from build123d import *

# Parameters (mm, degrees)
SKETCH1_W                      = 300
SKETCH1_H                      = 300
BOSS_EXTRUDE1_DEPTH            = 175
SHELL1_T                       = -10
CUT_EXTRUDE5_DEPTH             = 50
CUT_EXTRUDE6_START             = -50
CUT_EXTRUDE6_DEPTH             = 50
CUT_EXTRUDE7_REACH             = 380.319
SKETCH8_W                      = 150
SKETCH8_H                      = 20
CUT_EXTRUDE7_DIRECTION_2_DEPTH = 379.318648761


with BuildPart() as part:
    # Sketch1 → Boss-Extrude1 (new body)
    with BuildSketch(Plane(origin=(0, 0, 0), x_dir=(1, 0, 0), z_dir=(0, 1, 0))):
        Rectangle(SKETCH1_W, SKETCH1_H)
    extrude(amount=BOSS_EXTRUDE1_DEPTH)

    # Shell1
    shell1_openings = [part.faces().sort_by_distance(p)[0] for p in [
        (0, 175, 0),
    ]]
    offset(amount=SHELL1_T, openings=shell1_openings, kind=Kind.INTERSECTION)

    # Sketch4 → Cut-Extrude5 (cut)
    with BuildSketch(Plane.XY.offset(150)):
        with BuildLine():
            Line((0, 0), (75, 0))
            Line((75, 0), (75, 50))
            ThreePointArc((75, 50), (83.786796564, 71.213203436), (105, 80))
            Line((105, 80), (150, 80))
            Line((150, 80), (150, -5))
            Line((150, -5), (-150, -5))
            Line((-150, -5), (-150, 80))
            Line((-150, 80), (-105, 80))
            ThreePointArc((-105, 80), (-83.786796564, 71.213203436), (-75, 50))
            Line((-75, 50), (-75, 0))
            Line((-75, 0), (0, 0))
        make_face()
    extrude(amount=-CUT_EXTRUDE5_DEPTH, mode=Mode.SUBTRACT)

    # Sketch7 → Cut-Extrude6 (cut)
    with BuildSketch(Plane(origin=(0, 0, -150), x_dir=(-1, 0, 0), z_dir=(0, 0, -1)).offset(CUT_EXTRUDE6_START)):
        with BuildLine():
            Line((0, 0), (75, 0))
            Line((75, 0), (75, 50))
            ThreePointArc((75, 50), (83.786796564, 71.213203436), (105, 80))
            Line((105, 80), (150, 80))
            Line((150, 80), (150, -5))
            Line((150, -5), (-150, -5))
            Line((-150, -5), (-150, 80))
            Line((-150, 80), (-105, 80))
            ThreePointArc((-105, 80), (-83.786796564, 71.213203436), (-75, 50))
            Line((-75, 50), (-75, 0))
            Line((-75, 0), (0, 0))
        make_face()
    extrude(amount=CUT_EXTRUDE6_DEPTH, mode=Mode.SUBTRACT)

    # Sketch8 → Cut-Extrude7 (cut, up to next)
    with BuildSketch(Plane(origin=(150, 0, 0), x_dir=(0, 0, -1), z_dir=(1, 0, 0)), mode=Mode.PRIVATE) as cut_extrude7_sk1:
        with Locations((0, 100)):
            Rectangle(SKETCH8_W, SKETCH8_H)
    cut_extrude7_tool1 = extrude(cut_extrude7_sk1.sketch, amount=-CUT_EXTRUDE7_REACH, mode=Mode.PRIVATE) & part.part
    add(cut_extrude7_tool1.solids().sort_by_distance((150, 100, 0))[0], mode=Mode.SUBTRACT)

    # Sketch8 → Cut-Extrude7 direction 2 (cut)
    with BuildSketch(Plane(origin=(150, 0, 0), x_dir=(0, 0, -1), z_dir=(1, 0, 0))):
        with Locations((0, 100)):
            Rectangle(SKETCH8_W, SKETCH8_H)
    extrude(amount=CUT_EXTRUDE7_DIRECTION_2_DEPTH, mode=Mode.SUBTRACT)


solid = part.part
Source: CAD feature listing. Evaluate the final solid. Frame: model axes, mm. A direction names the side the tool comes from. Give positions to 0.01 mm unless a question says otherwise; leave off trailing zeros. Order: outer loops, then holes, each group sorted by start corner. A loop starts at its lowest first (then second) coordinate and runs counter-clockwise, first axis right, second up. Notation, with made-up numbers: (32, 53) -> (42, 53) arc R6 ccw to (42, 58) -> close; hole circle Ø9 at (46.5, 65.25). An arc over 180 degrees is marked (long way). Use a Markdown table: item, result.
1) Section query B-B, the plane y = 31.5. Return the cut outline in (x, z).
Answer list:
| item | result |
|---|---|
| outline | (-150, -100) -> (-140, -100) -> (-140, 100) -> (-150, 100) -> close; (-75, -150) -> (75, -150) -> (75, -140) -> (-75, -140) -> close; (-75, 140) -> (75, 140) -> (75, 150) -> (-75, 150) -> close; (140, -100) -> (150, -100) -> (150, 100) -> (140, 100) -> close |
2) Reachability of faces 1 (the flat face through (-2, 110, -140)), 2 (the flat face through (145, 110, 1)), 3 (the flat face through (142, 80, 136)) from +Z, -Z, +X, -X, +Y, -Y: full face, straight path, thin tool, end or side. Return the list, or none.
Answer list:
| item | result |
|---|---|
| face 1 | +Y |
| face 2 | +X |
| face 3 | +Z, +X, -Y |
3) Contact query for flat-ended pins moving along their axis: P1, Ø13.5, axis at x = 136, z = -135.5, coming from the -Y side; P2, Ø3, axis at x = 33, z = 47, coming from the +Y side. Output: stop coordinate, or through.
Answer list:
| item | result |
|---|---|
| P1 | y = 80 |
| P2 | y = 10 |
4) Section query D-D, the plane x = 128.5. Return the cut outline in (y, z).
Answer list:
| item | result |
|---|---|
| outline | (0, -100) -> (10, -100) -> (10, 100) -> (0, 100) -> close; (80, -150) -> (175, -150) -> (175, -140) -> (80, -140) -> close; (80, 140) -> (175, 140) -> (175, 150) -> (80, 150) -> close |
5) Section query C-C, the plane z = 1.5. Return the cut outline in (x, y).
Answer list:
| item | result |
|---|---|
| outline | (-150, 0) -> (150, 0) -> (150, 90) -> (140, 90) -> (140, 10) -> (-140, 10) -> (-140, 175) -> (-150, 175) -> close; (140, 110) -> (150, 110) -> (150, 175) -> (140, 175) -> close |
6) Section query A-A, the plane z = -120. Return the cut outline in (x, y).
Answer list:
| item | result |
|---|---|
| outline | (-150, 80) -> (-140, 80) -> (-140, 175) -> (-150, 175) -> close; (-75, 0) -> (75, 0) -> (75, 10) -> (-75, 10) -> close; (140, 80) -> (150, 80) -> (150, 175) -> (140, 175) -> close |
7) Mould query, pull axis Z, two halves, no side actions, for faces 4 (the flat face through (75, 8, 136)), 5 (the flat face through (-2, 10, -2)), 6 (the flat face through (-143, 25, 100)), 7 (the flat face through (-2, 106, -150)). Classes: +Z half, -Z half, draft (parallel to the pull), parting line (faces both ways), or undercut.
Answer list:
| item | result |
|---|---|
| face 4 | draft |
| face 5 | undercut |
| face 6 | +Z half |
| face 7 | -Z half |
8) Ray query, line 1 along Z through (x, y) = (72, 136); line 2 along Y through (x, z) = (-117.5, -25). Return the intervals inside material, ascending. Write a range as [from, to].
Answer list:
| item | result |
|---|---|
| line 1 | [-150, -140], [140, 150] |
| line 2 | [0, 10] |
